Autodesk Inventor part; units mm, degrees
ref_plane "Work Plane1" through (5, 0, 0) normal (0, -0.5, -0.866) x (1, 0, 0)
ref_plane "YZ Plane" through (0, 0, 0) normal (1, 0, 0) x (0, 1, 0)
ref_plane "XZ Plane" through (0, 0, 0) normal (0, 1, 0) x (-1, 0, 0)
sketch "Skizze1" plane through (0, 0, 0) normal (0, 0, 1) x (1, 0, 0)
  line L0 (0.5774, 0) -> (6.8333, 0)
  line L1 (10, 1.1547) -> (10, 2)
  line L2 (10, 2) -> (0, 2)
  line L3 (10, 1.1547) -> (7.5, 1.1547)
  line L4 (7.5, 1.1547) -> (6.8333, 0)
  line L5 (0, 1) -> (0.5774, 0)
  line L6 (0, -0.4) -> (0, 2.4)
  line L7 (0, 1) -> (0, 2)
  point P0 (0, 0)
  dimension "d0" = 2.5
  dimension "d1" = 60
  dimension "d2" = 4
  dimension "d3" = 2.3094
  dimension "d4" = 10
  dimension "d5" = 60
  dimension "d7" = 2
revolve "Körper" add sketch "Skizze1" angle 360 about axis through (0.5774, 0, 0) along (1, 0, 0)
sketch "Skizze2" plane through (10, 0, 0) normal (1, 0, 0) x (0, 0, -1)
  circle A0 centre (0, 0) radius 1.1547
  circle A1 centre (0, 0) radius 2
  line L0 (1.1547, 0) -> (0.5774, -1)
  line L1 (0.5774, -1) -> (-0.5774, -1)
  line L2 (-0.5774, -1) -> (-1.1547, 0)
  line L3 (-1.1547, 0) -> (-0.5774, 1)
  line L4 (-0.5774, 1) -> (0.5774, 1)
  line L5 (0.5774, 1) -> (1.1547, 0)
extrude "Loch" add sketch "Skizze2" against normal blind 2.5 contours L5 A0 | A0 L0 | L4 A0 | A0 L1 | L3 A0 | A0 L2
chamfer "Fase1" distance 1 angle 45 1 edges at (0, -2, 0) measured on face at (0, 1.6473, -0.1595)
thread "Gewinde"
chamfer "Fase2" distance 0.4294 angle 45 1 edges at (10, -2, 0) measured on face at (6.9998, 1.9741, -0.3208)
ref_plane "Work Plane1" through (5, 0, 0) normal (0, -0.5, -0.866) x (1, 0, 0)
equation "\"d0\" = INTI"
equation "\"d2\" = NND"
equation "\"d3\" = 1.1547 * SW"
equation "\"d4\" = NLG"
equation "\"d5\" = 0.5 * ANG"
equation "\"d7\" = SPD"
equation "\"d8\" = INTI"
equation "\"d10\" = -0.5 * SPD + 0.5 * NND"
equation "\"d11\" = FAWI"
equation "\"d33\" = -0.5 * SPD + 0.5 * NND"
equation "\"d14\" = NLG"
equation "\"d12\" = -0.5 * GD1 + 0.5 * NND"
equation "\"d13\" = FAWI"
equation "\"d34\" = -0.5 * GD1 + 0.5 * NND"
equation "\"NND\" = 4"
equation "\"NLG\" = 10"
equation "\"INTI\" = 2.5"
equation "\"FAWI\" = 45deg"
equation "\"SW\" = 2"
equation "\"GD1\" = THREADDIA - 1.2269 * PTC"
equation "\"ANG\" = 120deg"
equation "\"FAWI1\" = 45deg"
equation "\"SPD\" = 2"
equation "\"GUL\" = 0.61345 * PTC"
equation "\"TOA\" = 30deg"
equation "\"THREADDIA\" = 4"
equation "\"PTC\" = 0.7"
equation "\"GAL\" = 0.61345 * PTC"
equation "\"E0\" = 1.155 * SW"
properties part number "ISO 4029 - M4 x 10" material "Edelstahl, 440C"
Can you work these out from the model? Positions are in its coordinate system, mm. A direction names the side the tool comes from. Round coordinates to 2 decimals unless told otherwise and drop trailing zeros. Order: outer loops, then holes, each group sorted by start corner. A loop starts at its lowest first (then second) coordinate and runs counter-clockwise, first axis right, second up. Notation, with made-up numbers: (-8, -7.75) - (-2, -7.75) arc R28 ccw to (-2, 19.25) - close; hole circle Ø1 at (55.25, -16.75). An arc over 180 degrees is marked (long way). Answer in a Markdown table with one row per item.
(1) Please list where these lines run through material, in increasing order: L1, parallel to Y at x = 8.5, z = -0.1; L2, parallel to Y at x = 9.5, z = -1; L3, parallel to X at y = -1.1, z = -1.4. Write a range as from..to.
From the geometry:
| item | result |
|---|---|
| L1 | y = -2..-1, 1..2 |
| L2 | y = -1.73..-0.27, 0.27..1.73 |
| L3 | x = 0.78..9.79 |
(2) Suppose I cut it at A-A, the plane x = 8.75. Please give me the cut outline in (y, z).
From the geometry:
| item | result |
|---|---|
| outline | circle Ø4 at (0, 0); hole (-1, -0.58) - (0, -1.15) - (1, -0.58) - (1, 0.58) - (0, 1.15) - (-1, 0.58) - close |
(3) If we mould it in two halves opening along Y, with no side actions, what happens to faces 3 (the face through (5, 0, 2)), 4 (the face through (8.77, -0.49, -0.87))? For each: released by +Y, released by -Y, zero draft, split by the parting line, or undercut.
From the geometry:
| item | result |
|---|---|
| face 3 | split by the parting line |
| face 4 | undercut |
(4) Suppose I cut it at B-B, the plane x = 1.5. Please give me the cut outline in (y, z), plus the area to 3 significant figures.
From the geometry:
| item | result |
|---|---|
| outline | circle Ø4 at (0, 0) |
| area | 12.6 mm2 |
(5) Which directions (+Z, -Z, +X, -X, +Y, -Y) give clear straight access to the entire face, cutting with the end or side of a thin tool? Please do faces 1 (the face through (8.77, -0.51, 0.86)), 2 (the face through (0.477, -0.128, -0.117)).
From the geometry:
| item | result |
|---|---|
| face 1 | +X |
| face 2 | -X |
